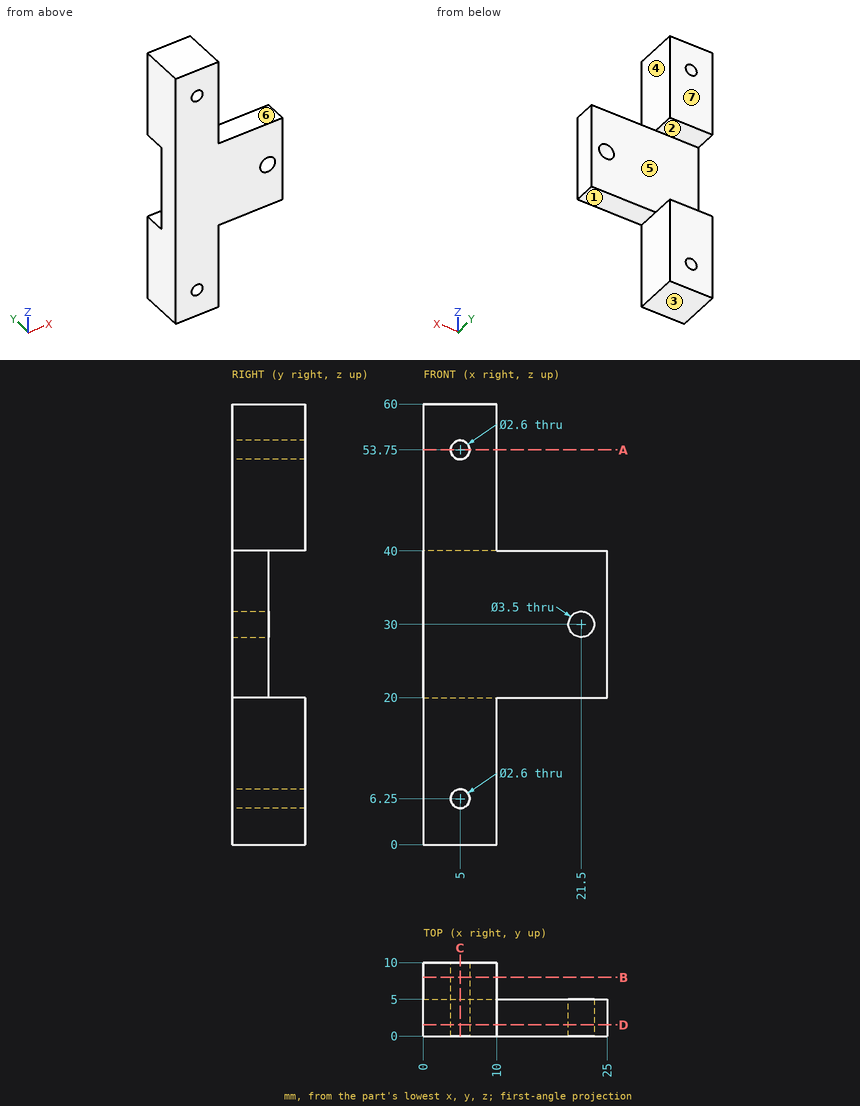
Geometry: see drawing. Coordinates: mm, zero at the bounding-box minimum. A direction names the side the tool comes from. Coordinates: 2 decimals unless noted, no trailing zeros. Loops run counter-clockwise (first coordinate to the right, second up) from the corner with the lowest first, then second, coordinate; pieces in that order, holes last.
Q1. Draft query along Z for the marked faces 5, 6 and 7. Return one class per face: +Z half, -Z half, draft (parallel to the pull), parting line (faces both ways), or undercut.
Q2. Material intervals for line 1 (Z direction, x = 5, y = 4.25); line 2 (Z direction, x = 5, y = 7); line 3 (Z direction, x = 21.5, y = 1.6), sorted ascending.
Q3. Cut plane B-B (y = 8). Output: boundary loops of the cut face in (x, z), then the cut area to 3 significant figures.
Q4. Cut plane D-D (y = 1.5). Output: boundary loops of the cut face in (x, z), then the cut area to 3 significant figures.
Q5. Cut plane C-C (x = 5). Output: boundary loops of the cut face in (y, z), then the cut area to 3 significant figures.
Q6. Set-up query: the marked faces 1, 2, 3 and 4. Return all of +Z, -Z, +X, -X, +Y, -Y with unobstructed straight access to the full face (end or side cutting, diameter ignored); none if empty.
Q7. Contact query for flat-ended pins moving along their axis: pin 1 (4 mm diameter, centred on x = 15.5, y = 3, fed in from -Z); pin 2 (1.5 mm diameter, centred on x = 21, y = 3, fed in from +Z); pin 3 (3 mm diameter, centred on y = 2.5, z = 14.5, fed in from +X). Output: stop coordinate, or through.
Q8. Cut plane A-A (z = 53.75). Output: boundary loops of the cut face in (x, y).
Working result:
1. face 5: undercut
1. face 6: +Z half
1. face 7: draft
2. line 1: z = 0 to 4.95, 7.55 to 52.45, 55.05 to 60
2. line 2: z = 0 to 4.95, 7.55 to 20, 40 to 52.45, 55.05 to 60
2. line 3: z = 20 to 28.25, 31.75 to 40
3. outline: (0, 0) - (10, 0) - (10, 20) - (0, 20) - close; (0, 40) - (10, 40) - (10, 60) - (0, 60) - close; hole circle Ø2.6 at (5, 6.25); hole circle Ø2.6 at (5, 53.75)
3. area: 389 mm2
4. outline: (0, 0) - (10, 0) - (10, 20) - (25, 20) - (25, 40) - (10, 40) - (10, 60) - (0, 60) - close; hole circle Ø2.6 at (5, 6.25); hole circle Ø2.6 at (5, 53.75); hole circle Ø3.5 at (21.5, 30)
4. area: 880 mm2
5. outline: (0, 0) - (10, 0) - (10, 4.95) - (0, 4.95) - close; (0, 7.55) - (10, 7.55) - (10, 20) - (5, 20) - (5, 40) - (10, 40) - (10, 52.45) - (0, 52.45) - close; (0, 55.05) - (10, 55.05) - (10, 60) - (0, 60) - close
5. area: 448 mm2
6. face 1: -Z, +X, +Y, -Y
6. face 2: +X, -X, +Y
6. face 3: -Z, +X, -X, +Y, -Y
6. face 4: +Z, +X, +Y, -Y
7. pin 1: stops at z = 20
7. pin 2: stops at z = 40
7. pin 3: stops at x = 10
8. outline: (0, 0) - (3.7, 0) - (3.7, 10) - (0, 10) - close; (6.3, 0) - (10, 0) - (10, 10) - (6.3, 10) - close
